The listing builds one solid part. Answer for the finished solid, in the listing's coordinates (mm). A direction names the side the tool comes from. Round coordinates to 2 decimals unless told otherwise and drop trailing zeros. Write each loop counter-clockwise with the first axis right and the second up, starting at its lowest first coordinate (ties: lowest second). Pieces come first, ordered by that corner, then holes.
(1) A cutting plane is placed at B-B, the plane y = -46.5. Give the vertices of the cut face in (x, z).
(2) Find the intervals of material crossed by probe 1 along X at (y, z) = (-58.5, 10.75); probe 2 along X at (y, z) = (11, 7.5); probe 3 along Y at (x, z) = (5, 4.25), in increasing order.
(3) A cutting plane is placed at A-A, the plane z = 2. Give the vertices of the cut face in (x, y).
(4) Each of these flat-tipped pins is pushed along its axis until it touches: pin 1 Ø5.5 at (x, z) = (14, 14.5) entering from -Y; pin 2 Ø1 at (x, z) = (10, 9.5) entering from +Y; pin 3 Ø10 at (x, y) = (12.5, -27.5) entering from -Z; pin 4 Ø3.5 at (x, y) = (-7, 12.12) entering from +Z. Where does it stop, or does it pass through?
(5) A cutting plane is placed at C-C, the plane y = 1. Give the number of separate pieces and of enclosed holes in the cut face, and give its area (3 significant figures).
(6) The mould has two halves that part along X. Classify faces 1 (the face through (-8.972, -57.37, 10.513)), 2 (the face through (-16.37, 0.1, 8.62)), 3 (the face through (-14.297, 13.986, 8.535)): +X half, -X half, draft (parallel to the pull), parting line (faces both ways), or undercut.
(7) For faces 4 (the face through (9.028, -57.37, 10.513)), 5 (the face through (-0.028, -62.526, 11.352)), 6 (the face through (-2, -61, 10)), determine the directions among +Z, -Z, +X, -X, +Y, -Y from which every point of the face is accessible in a straight line to the end or side of a thin tool.
from build123d import *

# Parameters (mm, degrees)
SKETCH7_W           = 40
SKETCH7_H           = 40
BOSS_EXTRUDE1_DEPTH = 11
LOFT1_START         = -20
LOFT1_DEPTH         = 40
SKETCH16_W          = 49.026286786
SKETCH16_H          = 65.242270374
SKETCH16_R          = 20
CUT_EXTRUDE3_DEPTH  = 6
SKETCH17_W          = 40
SKETCH17_H          = 5
BOSS_EXTRUDE5_DEPTH = 18
SKETCH10_R          = 2.25
CUT_EXTRUDE1_DEPTH  = 25
SKETCH11_W          = 4
SKETCH11_H          = 5
BOSS_EXTRUDE3_DEPTH = 8
SKETCH14_R          = 6
BOSS_EXTRUDE4_DEPTH = 4
LPATTERN1_COUNT     = 5
LPATTERN1_PITCH     = 9
SKETCH15_R          = 2
CUT_EXTRUDE2_DEPTH  = 83.194890505
CHAMFER1_SIZE       = 2.5
FILLET2_R           = 2
FILLET3_R           = 20


# Read off the part's stored shape, not the designer's step: Loft1
with BuildPart() as part:
    # Sketch7 → Boss-Extrude1 (new body)
    with BuildSketch(Plane.XY):
        Rectangle(SKETCH7_W, SKETCH7_H)
    extrude(amount=BOSS_EXTRUDE1_DEPTH)

    # Loft1 outline → Loft1 (add)
    with BuildSketch(Plane.YZ.offset(LOFT1_START)):
        with BuildLine():
            add(Edge.make_bspline(
                [(-38, 16), (-31.772819436, 16), (-26.227180564, 11), (-20, 11)],
                knots=[0, 0, 0, 0, 1, 1, 1, 1], degree=3))
            Line((-38, 16), (-38, 11))
            add(Edge.make_bspline(
                [(-38, 11), (-31.772819436, 11), (-26.227180564, 6), (-20, 6)],
                knots=[0, 0, 0, 0, 1, 1, 1, 1], degree=3))
            Line((-20, 6), (-20, 11))
        make_face()
    extrude(amount=LOFT1_DEPTH)

    # Sketch16 → Cut-Extrude3 (cut)
    with BuildSketch(Plane(origin=(0, 0, 0), x_dir=(-1, 0, 0), z_dir=(0, 0, -1))):
        Rectangle(SKETCH16_W, SKETCH16_H)
        Circle(SKETCH16_R, mode=Mode.SUBTRACT)
    extrude(amount=-CUT_EXTRUDE3_DEPTH, mode=Mode.SUBTRACT)

    # Sketch17 → Boss-Extrude5 (add)
    with BuildSketch(Plane(origin=(0, -38, 0), x_dir=(-1, 0, 0), z_dir=(0, -1, 0))):
        with Locations((0, -13.5)):
            Rectangle(SKETCH17_W, SKETCH17_H)
    extrude(amount=BOSS_EXTRUDE5_DEPTH)

    # Sketch10 → Cut-Extrude1 (cut)
    with BuildSketch(Plane.XY.offset(11)):
        with Locations((-7.00009521, 12.124420806)):
            Circle(SKETCH10_R)
        with Locations((6.99990479, 12.124420806)):
            Circle(SKETCH10_R)
        with Locations((13.99990479, 6.5153e-05)):
            Circle(SKETCH10_R)
        with Locations((6.99990479, -12.1242905)):
            Circle(SKETCH10_R)
        with Locations((-7.00009521, -12.1242905)):
            Circle(SKETCH10_R)
        with Locations((-14.00009521, 6.5153e-05)):
            Circle(SKETCH10_R)
    extrude(amount=-CUT_EXTRUDE1_DEPTH, mode=Mode.SUBTRACT)

    # Sketch11 → Boss-Extrude3 (add)
    with BuildSketch(Plane(origin=(0, -56, -3.472963553), x_dir=(1, 0, 0), z_dir=(0, 1, 0))):
        with Locations((-18, -16.972963553)):
            Rectangle(SKETCH11_W, SKETCH11_H)
    boss_extrude3 = extrude(amount=-BOSS_EXTRUDE3_DEPTH)

    # Sketch14 → Boss-Extrude4 (add)
    with BuildSketch(Plane(origin=(-16, 0, 0), x_dir=(0, 0, -1), z_dir=(1, 0, 0))):
        with Locations((-10, -64)):
            Circle(SKETCH14_R)
    boss_extrude4 = extrude(amount=-BOSS_EXTRUDE4_DEPTH)

    # LPattern1: Boss-Extrude3, Boss-Extrude4 ×5
    with Locations(*[(i * LPATTERN1_PITCH, 0, 0) for i in range(1, LPATTERN1_COUNT)]):
        add(boss_extrude3)
        add(boss_extrude4)

    # Sketch15 → Cut-Extrude2 (cut, through all)
    with BuildSketch(Plane.ZY.offset(20)):
        with Locations(Location((10, -64, 0), (0, 0, 270))):
            Circle(SKETCH15_R)
    extrude(amount=-CUT_EXTRUDE2_DEPTH, mode=Mode.SUBTRACT)

    # Chamfer1
    chamfer1_edges = [part.edges().sort_by_distance(p)[0] for p in [
        (4.74990479, 12.124420806, 11),
        (-9.25009521, 12.124420806, 11),
        (-16.25009521, 6.5153e-05, 11),
        (-9.25009521, -12.1242905, 11),
        (4.74990479, -12.1242905, 11),
        (11.74990479, 6.5153e-05, 11),
    ]]
    chamfer(chamfer1_edges, length=CHAMFER1_SIZE)

    # Fillet2
    fillet2_edges = [part.edges().sort_by_distance(p)[0] for p in [
        (-18, -58.083920217, 11),
        (-9, -58.083920217, 11),
        (0, -58.083920217, 11),
        (9, -58.083920217, 11),
        (18, -58.083920217, 11),
    ]]
    fillet(fillet2_edges, radius=FILLET2_R)

    # Fillet3
    fillet3_edges = [part.edges().sort_by_distance(p)[0] for p in [
        (20, 20, 8.5),
        (-20, 20, 8.5),
    ]]
    fillet(fillet3_edges, radius=FILLET3_R - 0.0001)  # a hair under: the kernel refuses the full size


solid = part.part
Solutions:
1. outline: (-20, 11) - (20, 11) - (20, 16) - (-20, 16) - close
2. probe 1: x = -20 to -16, -11 to -7, -2 to 2, 7 to 11, 16 to 20
2. probe 2: x = -16.7 to -8.95, -5.05 to 5.05, 8.95 to 16.7
2. probe 3: y = -19.36 to -13.16, -11.09 to 11.09, 13.16 to 19.36
3. outline: circle Ø40 at (0, 0); hole circle Ø4.5 at (-14, 0); hole circle Ø4.5 at (-7, -12.12); hole circle Ø4.5 at (-7, 12.12); hole circle Ø4.5 at (7, -12.12); hole circle Ø4.5 at (7, 12.12); hole circle Ø4.5 at (14, 0)
4. pin 1: stops at y = -69.4
4. pin 2: stops at y = 17.6
4. pin 3: stops at z = 6.25
4. pin 4: passes through
5. separate pieces: 3
5. enclosed holes: 0
5. area: 337 mm2
6. face 1: draft
6. face 2: undercut
6. face 3: -X half
7. face 4: -Z, +X, -X
7. face 5: +X, -X
7. face 6: +Z, -Z, -Y
